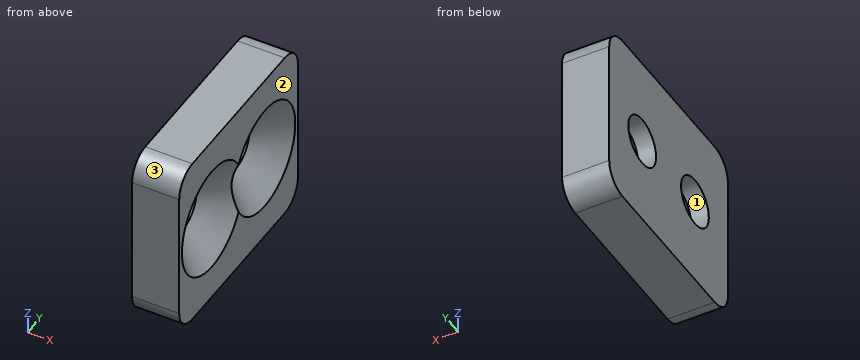
from build123d import *

# Parameters (mm, degrees)
SKETCH4_W           = 15
SKETCH4_H           = 18
SKETCH4_R           = 2.1
BOSS_EXTRUDE1_DEPTH = 4
FILLET1_R           = 2
CHAMFER1_SIZE       = 2.5


with BuildPart() as part:
    # Sketch4 → Boss-Extrude1 (new body)
    with BuildSketch(Plane(origin=(0, 0, 0), x_dir=(0, 0, -1), z_dir=(1, 0, 0))):
        Rectangle(SKETCH4_W, SKETCH4_H)
        with Locations((0, 4)):
            Circle(SKETCH4_R, mode=Mode.SUBTRACT)
        with Locations((0, -4)):
            Circle(SKETCH4_R, mode=Mode.SUBTRACT)
    extrude(amount=BOSS_EXTRUDE1_DEPTH)

    # Fillet1
    fillet1_edges = [part.edges().sort_by_distance(p)[0] for p in [
        (2, -9, -7.5),
        (2, -9, 7.5),
        (2, 9, 7.5),
        (2, 9, -7.5),
    ]]
    fillet(fillet1_edges, radius=FILLET1_R)

    # Chamfer1
    # the kernel refuses this chamfer: 2.5 mm, written as the material it takes off along each edge
    with BuildSketch(Plane(origin=(4, 4, 0), x_dir=(0, 0, -1), z_dir=(0, -1, 0))) as chamfer1_piece_1:
        Polygon((2.1 + CHAMFER1_SIZE, 0), (2.1, -CHAMFER1_SIZE), (2.1, 0), align=None)
    revolve(axis=Axis((4, 4, 0), (1, 0, 0)), mode=Mode.SUBTRACT)
    with BuildSketch(Plane(origin=(4, -4, 0), x_dir=(0, 0, -1), z_dir=(0, -1, 0))) as chamfer1_piece_2:
        Polygon((2.1 + CHAMFER1_SIZE, 0), (2.1, -CHAMFER1_SIZE), (2.1, 0), align=None)
    revolve(axis=Axis((4, -4, 0), (1, 0, 0)), mode=Mode.SUBTRACT)


solid = part.part
Here's how the part is built. I have some questions about the finished solid (model axes, mm). Face numbers are marked on the shaded views. Round coordinates to 2 decimals unless told otherwise and drop trailing zeros. Write each loop counter-clockwise with the first axis right and the second up, starting at its lowest first coordinate (ties: lowest second). Pieces come first, ordered by that corner, then holes.
1. Will this pin go through, and if not, where does the flat tip stop? pin 1 Ø4 at (y, z) = (4, 0) entering from -X.
2. If we mould it in two halves opening along Y, with no side actions, what happens to the marked faces 1, 2 and 3? For each: released by +Y, released by -Y, zero draft, split by the parting line, or undercut.
3. Suppose I cut it at C-C (x = 3.3). List the corners of the cut face in (y, z) for me.
4. I need wall thicknesses on L1, parallel to Y at x = 0.8, z = 0; L2, parallel to Y at x = 3.25, z = 3; L3, parallel to Z at x = 3.05, y = -3.75. Which ranges of each line are inside material? Lowest first, please.
5. Suppose I cut it at B-B (z = 0). List the corners of the cut face in (x, y) for me, and give its area (3 significant figures).
6. Suppose I cut it at A-A (y = -4). List the corners of the cut face in (x, z) for me, and give its area (4 significant figures).
7. Suppose I cut it at D-D (x = 0.3). List the corners of the cut face in (y, z) for me.
Answer sheet:
1. pin 1: passes through
2. face 1: undercut
2. face 2: zero draft
2. face 3: released by -Y
3. outline: (-9, -5.5) arc R2 ccw to (-7, -7.5) - (7, -7.5) arc R2 ccw to (9, -5.5) - (9, 5.5) arc R2 ccw to (7, 7.5) - (-7, 7.5) arc R2 ccw to (-9, 5.5) - close; hole circle Ø7.8 at (-4, 0); hole circle Ø7.8 at (4, 0)
4. L1: y = -9 to -6.1, -1.9 to 1.9, 6.1 to 9
4. L2: y = -9 to -6.41, -1.59 to 1.59, 6.41 to 9
4. L3: z = -7.5 to -3.64, 3.64 to 7.5
5. outline: (0, -9) - (4, -9) - (4, -8.6) - (1.5, -6.1) - (0, -6.1) - close; (0, -1.9) - (1.5, -1.9) - (3.4, 0) - (1.5, 1.9) - (0, 1.9) - close; (0, 6.1) - (1.5, 6.1) - (4, 8.6) - (4, 9) - (0, 9) - close
5. area: 26.3 mm2
6. outline: (0, -7.5) - (4, -7.5) - (4, -4.6) - (1.5, -2.1) - (0, -2.1) - close; (0, 2.1) - (1.5, 2.1) - (4, 4.6) - (4, 7.5) - (0, 7.5) - close
6. area: 36.95 mm2
7. outline: (-9, -5.5) arc R2 ccw to (-7, -7.5) - (7, -7.5) arc R2 ccw to (9, -5.5) - (9, 5.5) arc R2 ccw to (7, 7.5) - (-7, 7.5) arc R2 ccw to (-9, 5.5) - close; hole circle Ø4.2 at (-4, 0); hole circle Ø4.2 at (4, 0)
